Input: dimensioned drawing with shaded views. Units: mm. Origin: part minimum x, y, z. A direction names the side the tool comes from. Round coordinates to 2 decimals unless told otherwise and drop trailing zeros. Write each loop counter-clockwise with the first axis right and the second up, starting at its lowest first coordinate (ties: lowest second). Pieces come first, ordered by that corner, then holes. Notation, with made-up numbers: (41.5, -37.75) -> (88.5, -37.75) arc R18 cw to (88.5, -13.75) -> close; hole circle Ø11 at (44, 30.25). An arc over 180 degrees is marked (long way). Return JSON: item names as keys, results as strings. Group by question number.
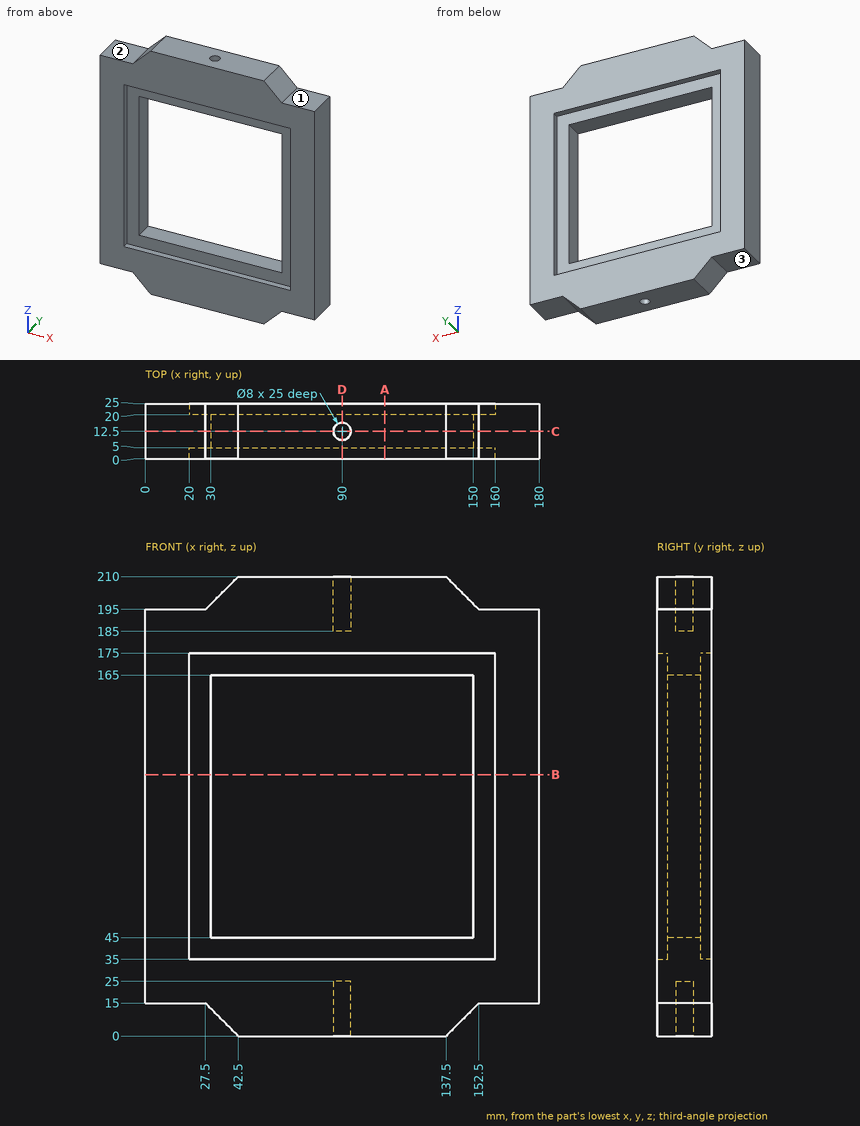
Item 1: Material intervals for probe 1 along Z at (x, y) = (117, 17.5); probe 2 along Y at (x, z) = (90, 12.25); probe 3 along Z at (x, y) = (54.5, 4), sorted ascending.
Item 2: Set-up query: the marked faces 1, 2 and 3. Return all of +Z, -Z, +X, -X, +Y, -Y with unobstructed straight access to the full face (end or side cutting, diameter ignored); none if empty.
Item 3: Cut plane D-D on x = 90. Output: boundary loops of the cut face in (y, z).
Item 4: First-contact query: pin 1 Ø7.5 at (x, y) = (167.5, 8.5) entering from +Z; pin 2 Ø7.5 at (x, y) = (11.5, 17) entering from -Z. Flat tips, straight axial feed; report the tip coordinate or a pass-through.
Item 5: Cut plane B-B on z = 119.5. Output: boundary loops of the cut face in (x, y), and give its area (3 significant figures).
Item 6: Cut plane A-A on x = 109.5. Output: boundary loops of the cut face in (y, z), and give its area (3 significant figures).
Item 7: Cut plane C-C on y = 12.5. Output: boundary loops of the cut face in (x, z).
Here are the results:
{
 "1": {"probe 1": "z = 0 to 45, 165 to 210", "probe 2": "y = 0 to 8.5, 16.5 to 25", "probe 3": "z = 0 to 35, 175 to 210"},
 "2": {"face 1": "+Z, +X, +Y, -Y", "face 2": "+Z, -X, +Y, -Y", "face 3": "-Z, -X, +Y, -Y"},
 "3": {"outline": "(0, 0) -> (8.5, 0) -> (8.5, 25) -> (16.5, 25) -> (16.5, 0) -> (25, 0) -> (25, 35) -> (20, 35) -> (20, 45) -> (5, 45) -> (5, 35) -> (0, 35) -> close; (0, 175) -> (5, 175) -> (5, 165) -> (20, 165) -> (20, 175) -> (25, 175) -> (25, 210) -> (16.5, 210) -> (16.5, 185) -> (8.5, 185) -> (8.5, 210) -> (0, 210) -> close"},
 "4": {"pin 1": "stops at z = 195", "pin 2": "stops at z = 15"},
 "5": {"outline": "(0, 0) -> (20, 0) -> (20, 5) -> (30, 5) -> (30, 20) -> (20, 20) -> (20, 25) -> (0, 25) -> close; (150, 5) -> (160, 5) -> (160, 0) -> (180, 0) -> (180, 25) -> (160, 25) -> (160, 20) -> (150, 20) -> close", "area": "1,300 mm^2"},
 "6": {"outline": "(0, 0) -> (25, 0) -> (25, 35) -> (20, 35) -> (20, 45) -> (5, 45) -> (5, 35) -> (0, 35) -> close; (0, 175) -> (5, 175) -> (5, 165) -> (20, 165) -> (20, 175) -> (25, 175) -> (25, 210) -> (0, 210) -> close", "area": "2,050 mm^2"},
 "7": {"outline": "(0, 15) -> (27.5, 15) -> (42.5, 0) -> (86, 0) -> (86, 25) -> (94, 25) -> (94, 0) -> (137.5, 0) -> (152.5, 15) -> (180, 15) -> (180, 195) -> (152.5, 195) -> (137.5, 210) -> (94, 210) -> (94, 185) -> (86, 185) -> (86, 210) -> (42.5, 210) -> (27.5, 195) -> (0, 195) -> close; hole (30, 45) -> (150, 45) -> (150, 165) -> (30, 165) -> close"}
}
